Source: three-view drawing plus pictorial views. Frame: mm from the lowest corner of the part. A direction names the side the tool comes from. Coordinates: 2 decimals unless noted, no trailing zeros. Write each loop counter-clockwise with the first axis right and the second up, starting at its lowest first coordinate (ties: lowest second). Pieces come first, ordered by that corner, then holes. Notation, with made-up numbers: (36, 78) - (78, 78) arc R19 cw to (78, 83) - close; hole circle Ø4 at (-10, 67.5). An arc over 180 degrees is marked (long way). Put each result on its own line as item: value. Start each with the question number.
1. Cut plane D-D, the plane z = 8.5. Return loops of the section in (x, y), and give its area (3 significant figures).
2. Line query: line 1 (Z direction, x = 8.3, y = 1.8); line 2 (Y direction, x = 11, z = 9.25); line 3 (X direction, y = 7.5, z = 6). Output: solid intervals per line, ascending.
3. Cut plane C-C, the plane z = 5. Return loops of the section in (x, y).
4. Cut plane A-A, the plane y = 11.7. Return loops of the section in (x, z).
5. Access query for the marked faces 5 and 6. Directions: +Z, -Z, +X, -X, +Y, -Y. A direction counts if a zero-diameter tool reaches every point of the face in a straight line with its end or side. Return the directions, or none.
6. Cut plane B-B, the plane x = 8.3. Return loops of the section in (y, z), and give its area (3 significant figures).
7. Pin query (flat end, axial travel): pin 1 (5 mm diameter, centred on y = 11.7, z = 5, fed in from -X); pin 2 (2 mm diameter, centred on y = 8.5, z = 4.5, fed in from -X). Return the tip coordinate at first contact, or that it passes through.
8. Pull-direction query (X, two-part tool) for the marked faces 1, 2, 3 and 4; classes: released by +X, released by -X, zero draft, split by the parting line, or undercut.
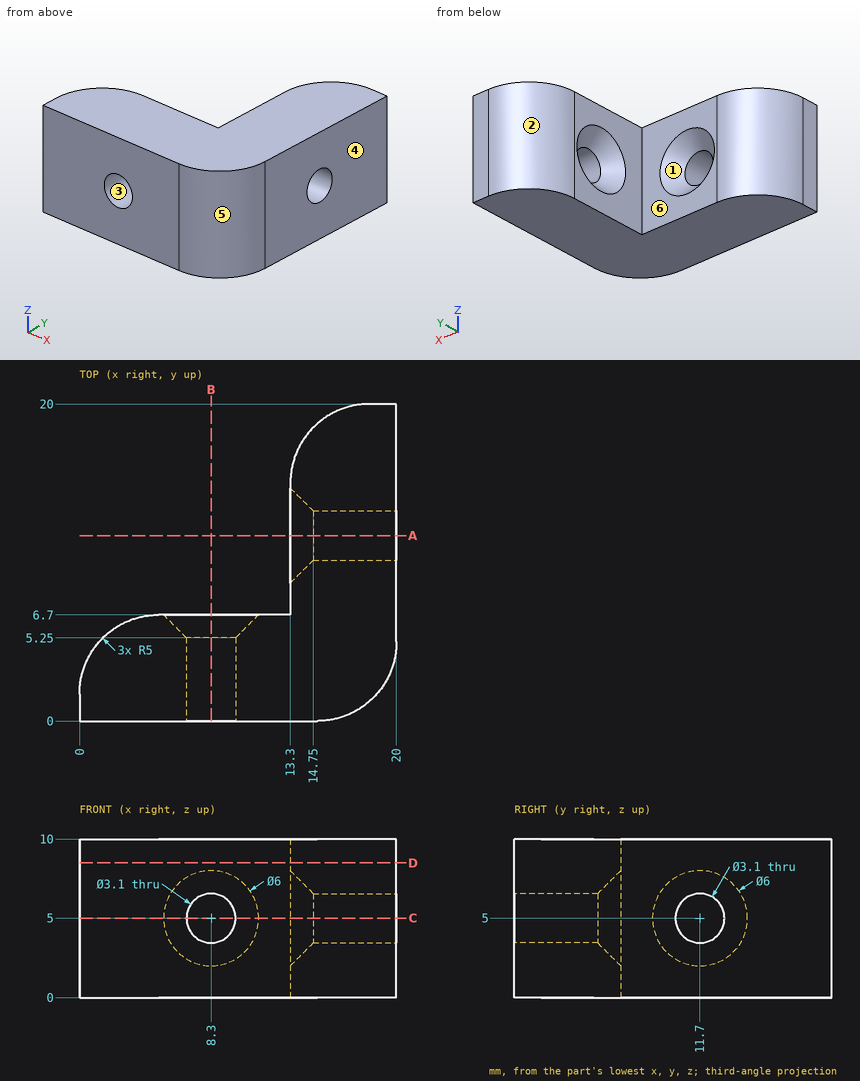
Report:
1. outline: (0, 0) - (15, 0) arc R5 ccw to (20, 5) - (20, 20) - (18.3, 20) arc R5 ccw to (13.3, 15) - (13.3, 6.7) - (5, 6.7) arc R5 ccw to (0, 1.7) - close
1. area: 207 mm^2
2. line 1: z = 0 to 3.45, 6.55 to 10
2. line 2: y = 0 to 6.7
2. line 3: x = 13.3 to 20
3. outline: (0, 0) - (6.75, 0) - (6.75, 5.25) - (5.3, 6.7) - (5, 6.7) arc R5 ccw to (0, 1.7) - close; (9.85, 0) - (15, 0) arc R5 ccw to (20, 5) - (20, 10.15) - (14.75, 10.15) - (13.3, 8.7) - (13.3, 6.7) - (11.3, 6.7) - (9.85, 5.25) - close; (13.3, 14.7) - (14.75, 13.25) - (20, 13.25) - (20, 20) - (18.3, 20) arc R5 ccw to (13.3, 15) - close
4. outline: (13.3, 0) - (20, 0) - (20, 3.45) - (14.75, 3.45) - (13.3, 2) - close; (13.3, 8) - (14.75, 6.55) - (20, 6.55) - (20, 10) - (13.3, 10) - close
5. face 5: +Z, -Z, +X, -Y
5. face 6: +Z, -Z, -X, +Y
6. outline: (0, 0) - (6.7, 0) - (6.7, 2) - (5.25, 3.45) - (0, 3.45) - close; (0, 6.55) - (5.25, 6.55) - (6.7, 8) - (6.7, 10) - (0, 10) - close
6. area: 44.1 mm^2
7. pin 1: stops at x = 13.8
7. pin 2: stops at x = 13.3
8. face 1: undercut
8. face 2: released by -X
8. face 3: undercut
8. face 4: released by +X
